Build history of the part. All positions in model axes, mm. Round coordinates to 2 decimals unless told otherwise and drop trailing zeros. Order: outer loops, then holes, each group sorted by start corner. A loop starts at its lowest first (then second) coordinate and runs counter-clockwise, first axis right, second up. Notation, with made-up numbers: (25.25, -14.75) -> (59.25, -14.75) arc R20 cw to (59.25, -8.75) -> close; hole circle Ø5 at (21, -19.5). An arc over 180 degrees is marked (long way). Answer as a JSON object with one key per item and string values.
from build123d import *

# Parameters (mm, degrees)
SKETCH1_R           = 14.224
SKETCH1_R_2         = 7.874
BOSS_EXTRUDE1_DEPTH = 96.52
FILLET1_R           = 1.27
FILLET2_R           = 0.762


with BuildPart() as part:
    # Sketch1 → Boss-Extrude1 (new body)
    with BuildSketch(Plane.XY):
        with Locations(Location((0, 0, 0), (0, 0, 180))):
            Circle(SKETCH1_R)
        with Locations(Location((0, 0, 0), (0, 0, 180))):
            Circle(SKETCH1_R_2, mode=Mode.SUBTRACT)
    extrude(amount=BOSS_EXTRUDE1_DEPTH)

    # Fillet1
    fillet1_edges = [part.edges().sort_by_distance(p)[0] for p in [
        (14.224, 0, 0),
        (14.224, 0, 96.52),
    ]]
    fillet(fillet1_edges, radius=FILLET1_R)

    # Fillet2
    fillet2_edges = [part.edges().sort_by_distance(p)[0] for p in [
        (7.874, 0, 0),
        (7.874, 0, 96.52),
    ]]
    fillet(fillet2_edges, radius=FILLET2_R)


solid = part.part
1) Probe L1, parallel to Y at x = 0, z = 41; L2, parallel to X at y = -2.25, z = 87; L3, parallel to Y at x = -5, z = 39. List the from-to ranges inside material, lowest first. Write a range as from..to.
Checked values:
{"L1": "y = -14.22..-7.87, 7.87..14.22", "L2": "x = -14.04..-7.55, 7.55..14.04", "L3": "y = -13.32..-6.08, 6.08..13.32"}
2) Pull direction Y, two halves, no side cores. Call faces 1 (the face through (-2.7, 8.5, 96.52)), 2 (the face through (3.083, 13.886, 47.602)), 3 (the face through (1.707, 7.687, 47.595)): pulls with the +Y half, pulls with the -Y half, needs draft (parallel to the pull), parting line crosses it, or undercut.
Checked values:
{"face 1": "needs draft", "face 2": "parting line crosses it", "face 3": "undercut"}
3) Cut at C-C, the plane z = 60.5. Give the cut face in (x, y).
Checked values:
{"outline": "circle Ø28.45 at (0, 0); hole circle Ø15.75 at (0, 0)"}
4) Cut at A-A, the plane y = 0. Give the cut face in (x, z), plus the area to 3 significant figures.
Checked values:
{"outline": "(-14.22, 1.27) arc R1.27 ccw to (-12.95, 0) -> (-8.64, 0) arc R0.76 ccw to (-7.87, 0.76) -> (-7.87, 95.76) arc R0.76 ccw to (-8.64, 96.52) -> (-12.95, 96.52) arc R1.27 ccw to (-14.22, 95.25) -> close; (7.87, 0.76) arc R0.76 ccw to (8.64, 0) -> (12.95, 0) arc R1.27 ccw to (14.22, 1.27) -> (14.22, 95.25) arc R1.27 ccw to (12.95, 96.52) -> (8.64, 96.52) arc R0.76 ccw to (7.87, 95.76) -> close", "area": "1,220 mm²"}
5) Flat gauge pins, fed straight in: pin 1 Ø4 at (x, y) = (7.5, 3) entering from -Z; pin 2 Ø12 at (x, z) = (11, 29) entering from +Y; pin 3 Ø1.5 at (y, z) = (3.5, 58) entering from -X; pin 4 Ø4 at (x, z) = (-11.5, 81) entering from +Y. Where does each tip first touch, or does it go through?
Checked values:
{"pin 1": "stops at z = 0", "pin 2": "stops at y = 13.32", "pin 3": "stops at x = -13.96", "pin 4": "stops at y = 10.59"}
